Build history of the part. All positions in model axes, mm. Face numbers are marked on the shaded views. A direction names the side the tool comes from. Give positions to 0.01 mm unless a question says otherwise; leave off trailing zeros. Order: outer loops, then holes, each group sorted by start corner. A loop starts at its lowest first (then second) coordinate and runs counter-clockwise, first axis right, second up. Notation, with made-up numbers: M -17.5,64 L 35.5,64 A20 cw 35.5,85 Z; hole C 76,23 d4. An arc over 180 degrees is marked long. One line per item, written item: value.
from build123d import *

# Parameters (mm, degrees)
F0_W     = 52.326445
F0_H     = 54.046918
F1_DEPTH = 38.1
F3_D     = 25.4
F4_W     = 25.4
F4_H     = 19.942893
F4_W_2   = 0.366597
F4_H_2   = 0.366597
F5_DEPTH = 12.7
F6_R     = 8.487976
F6_R_2   = 1.067547
F7_DEPTH = 6.35


with BuildPart() as f1:
    # F0 (on Front) → F1 (new body)
    with BuildSketch(Plane.XZ):
        with Locations((-26.163222, 27.023459)):
            Rectangle(F0_W, F0_H)
    extrude(amount=F1_DEPTH)

    # F3 (through all)
    with Locations(Plane.XY.offset(54.046918)):
        with Locations((-27.433222, -18.808095)):
            Hole(F3_D / 2)

    # F4 (on face) → F5 (join)
    with BuildSketch(Plane.XZ.offset(38.1)):
        with Locations((-23.617967, 28.19657)):
            Rectangle(F4_W, F4_H)
        with Locations((-30.049153, 25.520409)):
            Rectangle(F4_W_2, F4_H_2, mode=Mode.SUBTRACT)
    extrude(amount=F5_DEPTH)

    # F6 (on face) → F7 (join)
    with BuildSketch(Plane.YZ):
        with Locations((-17.562686, 24.310639)):
            Circle(F6_R)
        with Locations((-19.908907, 29.516321)):
            Circle(F6_R_2, mode=Mode.SUBTRACT)
    extrude(amount=F7_DEPTH)


solid = f1.part
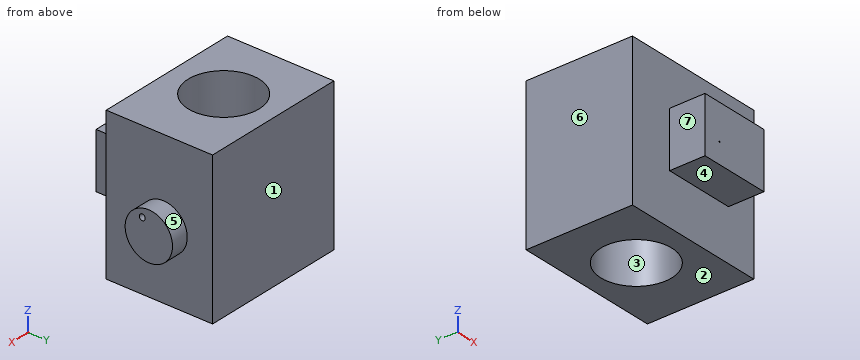
1) Saw through at D-D, the plane x = -13.5. Write the cut outline in (y, z).
Check values:
outline: M -50.8,18.23 L -38.1,18.23 L -38.1,0 L 0,0 L 0,54.05 L -38.1,54.05 L -38.1,38.17 L -50.8,38.17 Z
2) Pin check, flat tips, straight feed: pin 1 (6.5 mm diameter, centred on x = -26.5, y = -42.5, fed in from -Z); pin 2 (4 mm diameter, centred on y = -42.5, z = 25, fed in from +X); pin 3 (12 mm diameter, centred on y = -8.5, z = 39.5, fed in from +X). Stop position of each tip, or through.
Check values:
pin 1: z = 18.23
pin 2: x = -10.92
pin 3: x = 0
3) Tool access for the marked faces 4, 5, 6 and 7: list every direction of +Z, -Z, +X, -X, +Y, -Y with a clear straight run to the whole face (end or side of a thin tool).
Check values:
face 4: -Z, +X, -X, -Y
face 5: +X
face 6: +Z, -Z, -X, +Y, -Y
face 7: +Z, -Z, -X, -Y
4) Saw through at C-C, the plane y = -39. Write the cut outline in (x, z), then the cut area to 3 significant figures.
Check values:
outline: M -36.32,18.23 L -10.92,18.23 L -10.92,38.17 L -36.32,38.17 Z; hole M -30.23,25.34 L -29.87,25.34 L -29.87,25.7 L -30.23,25.7 Z
area: 506 mm^2
5) Drill centre lines: probe 1 along X at (y, z) = (-37, 18); probe 2 along Y at (x, z) = (-1.5, 28.5); probe 3 along Y at (x, z) = (-33.5, 33.5). Where is each one in solid material? Low to high. Write a range as from..to.
Check values:
probe 1: -52.33..0
probe 2: -38.1..0
probe 3: -50.8..-29.97, -7.65..0
6) Saw through at B-B, the plane z = 23. Write the cut outline in (x, y).
Check values:
outline: M -52.33,-38.1 L -36.32,-38.1 L -36.32,-50.8 L -10.92,-50.8 L -10.92,-38.1 L 0,-38.1 L 0,-25.95 L 6.35,-25.95 L 6.35,-9.18 L 0,-9.18 L 0,0 L -52.33,0 Z; hole C -27.43,-18.81 d25.4
7) Mould opens along Y. For the marked faces 1, 2 and 3 say: released by +Y, released by -Y, zero draft, split by the parting line, or undercut.
Check values:
face 1: released by +Y
face 2: zero draft
face 3: undercut
8) Saw through at A-A, the plane x = -26. Write the cut outline in (y, z), then the cut area to 3 significant figures.
Check values:
outline: M -50.8,18.23 L -38.1,18.23 L -38.1,0 L -31.43,0 L -31.43,54.05 L -38.1,54.05 L -38.1,38.17 L -50.8,38.17 Z; M -6.19,0 L 0,0 L 0,54.05 L -6.19,54.05 Z
area: 948 mm^2
